Geometry check sheet. Reference: the model listing, model coordinates, mm. A direction names the side the tool comes from. Round coordinates to 2 decimals unless told otherwise and drop trailing zeros. Order: outer loops, then holes, each group sorted by start corner. A loop starts at its lowest first (then second) coordinate and runs counter-clockwise, first axis right, second up. Notation, with made-up numbers: (37, 50.5) -> (79, 50.5) arc R35 cw to (79, 88.5) -> close; hole circle Ø9 at (-18, 29). An arc over 180 degrees is marked (long way). Use a Markdown table: item, result. Add a question column.
Item 1: Set-up check for faces 1 (the flat face through (35, 2, -32)), 2 (the flat face through (165, 2, 2)), 3 (the flat face through (182, 2, -37.3)), 4 (the flat face through (3, 2, -27.3)): record each of +Z, -Z, +X, -X, +Y, -Y from which the full face is reachable in a straight line by a thin tool's end or side.
Item 2: Sectioned sample at C-C, the plane x = 96. Record the cut outline in (y, z).
Item 3: Material ranges on probe 1 along X at (y, z) = (2.2, -10); probe 2 along X at (y, z) = (3.7, -12); probe 3 along X at (y, z) = (1.85, -21.15), recorded low to high. Write a range as [from, to].
Item 4: Sectioned sample at B-B, the plane y = 3.85. State how many separate pieces and enclosed holes the cut face has, and give its area (3 significant figures).
Item 5: Mould release check, pull along X, two halves, no side actions. Record for faces 5 (the flat face through (40, 2, -10)), 6 (the flat face through (2, 2, -37.3)), 7 (the cylindrical face through (183.987, 2.465, -21.345)), 8 (the cylindrical face through (183, 2, 9)): pulls with the +X half, pulls with the -X half, needs draft (parallel to the pull), parting line crosses it, or undercut.
Item 6: Gauge pin test, flat ends, axial feed: pin 1 Ø2.5 at (y, z) = (2.5, -33.5) entering from -X; pin 2 Ø1.5 at (y, z) = (1.5, -33.5) entering from +X; pin 3 Ø1.5 at (x, y) = (183, 3) entering from +Z; pin 4 Ø1.8 at (x, z) = (49, -32.3) entering from +Y. Record the tip position at first contact, or that the pin passes through.
Item 7: Sectioned sample at A-A, the plane z = -29. Record the cut outline in (x, y), and give its area (3 significant figures).
from build123d import *

# Parameters (mm, degrees)
SKETCH_1_R      = 1.5
SKETCH_1_W      = 5
SKETCH_1_H      = 10
EXTRUDE_1_DEPTH = 5


with BuildPart() as part:
    # 草图1 → 凸台-拉伸1 (new body)
    with BuildSketch(Plane(origin=(0, 0, 0), x_dir=(1, 0, 0), z_dir=(0, 1, 0))):
        with BuildLine():
            Line((0, 0), (0, -5))
            ThreePointArc((0, -5), (1.464466094, -8.535533906), (5, -10))
            Line((5, -10), (15, -10))
            ThreePointArc((15, -10), (18.535533906, -8.535533906), (20, -5))
            Line((20, -5), (20, 0))
            Line((20, 0), (165, 0))
            Line((165, 0), (165, -5))
            ThreePointArc((165, -5), (166.464466094, -8.535533906), (170, -10))
            Line((170, -10), (180, -10))
            ThreePointArc((180, -10), (183.535533906, -8.535533906), (185, -5))
            Line((185, -5), (185, 0))
            Line((185, 0), (185, 5))
            Line((185, 5), (180, 5))
            Line((180, 5), (180, 15))
            Line((180, 15), (185, 15))
            Line((185, 15), (185, 27.3))
            Line((185, 27.3), (180, 27.3))
            Line((180, 27.3), (180, 37.3))
            Line((180, 37.3), (185, 37.3))
            Line((185, 37.3), (185, 42.3))
            Line((185, 42.3), (0, 42.3))
            Line((0, 42.3), (0, 37.3))
            Line((0, 37.3), (5, 37.3))
            Line((5, 37.3), (5, 27.3))
            Line((5, 27.3), (0, 27.3))
            Line((0, 27.3), (0, 15))
            Line((0, 15), (5, 15))
            Line((5, 15), (5, 5))
            Line((5, 5), (0, 5))
            Line((0, 5), (0, 0))
        make_face()
        with Locations(Location((26, 32.3, 0), (0, 0, 270))):
            Circle(SKETCH_1_R, mode=Mode.SUBTRACT)
        with Locations(Location((49, 32.3, 0), (0, 0, 270))):
            Circle(SKETCH_1_R, mode=Mode.SUBTRACT)
        with Locations(Location((26, 10, 0), (0, 0, 270))):
            Circle(SKETCH_1_R, mode=Mode.SUBTRACT)
        with Locations(Location((49, 10, 0), (0, 0, 270))):
            Circle(SKETCH_1_R, mode=Mode.SUBTRACT)
        with Locations(Location((2.5, 21.15, 0), (0, 0, 270))):
            Circle(SKETCH_1_R, mode=Mode.SUBTRACT)
        with Locations(Location((182.5, 21.15, 0), (0, 0, 270))):
            Circle(SKETCH_1_R, mode=Mode.SUBTRACT)
        with Locations(Location((37.5, 21.15, 0), (0, 0, 270))):
            Circle(SKETCH_1_R, mode=Mode.SUBTRACT)
        with Locations((37.5, 32.3)):
            Rectangle(SKETCH_1_W, SKETCH_1_H, mode=Mode.SUBTRACT)
        with Locations((37.5, 10)):
            Rectangle(SKETCH_1_W, SKETCH_1_H, mode=Mode.SUBTRACT)
    extrude(amount=EXTRUDE_1_DEPTH)


solid = part.part
Found:
| question | item | result |
|---|---|---|
| 1 | face 1 | +Y, -Y |
| 1 | face 2 | +Z, +Y, -Y |
| 1 | face 3 | +X, +Y, -Y |
| 1 | face 4 | -X, +Y, -Y |
| 2 | outline | (0, -42.3) -> (5, -42.3) -> (5, 0) -> (0, 0) -> close |
| 3 | probe 1 | x = [5, 24.5], [27.5, 35], [40, 47.5], [50.5, 180] |
| 3 | probe 2 | x = [5, 35], [40, 180] |
| 3 | probe 3 | x = [0, 1], [4, 36], [39, 181], [184, 185] |
| 4 | separate pieces | 1 |
| 4 | enclosed holes | 9 |
| 4 | area | 7,850 mm2 |
| 5 | face 5 | undercut |
| 5 | face 6 | needs draft |
| 5 | face 7 | undercut |
| 5 | face 8 | pulls with the +X half |
| 6 | pin 1 | stops at x = 5 |
| 6 | pin 2 | stops at x = 180 |
| 6 | pin 3 | stops at z = 9.47 |
| 6 | pin 4 | passes through |
| 7 | outline | (5, 0) -> (35, 0) -> (35, 5) -> (5, 5) -> close; (40, 0) -> (180, 0) -> (180, 5) -> (40, 5) -> close |
| 7 | area | 850 mm2 |
